Autodesk Fusion 360 part; units mm, degrees
sketch "5.5 drilling alignment tool" plane through (0, 0, 0) normal (0, 1, 0) x (1, 0, 0)
  circle A0 centre (0, 0) radius 2.75
  circle A1 centre (0, 0) radius 4.35
  circle A2 centre (0, 0) radius 21
  line L0 (0, 0) -> (0, 30.5486) construction
  line L1 (0, 0) -> (37.4223, 0) construction
  line L2 (5, 0.7) -> (19, 0.7)
  line L3 (19, 0.7) -> (19, -0.7)
  line L4 (19, -0.7) -> (5, -0.7)
  line L5 (5, -0.7) -> (5, 0.7)
  dimension "d1" = 5.5
  dimension "d2" = 1.6
  dimension "d3" = 42
  dimension "d12" = 5
  dimension "d13" = 14
  dimension "d14" = 1.4
extrude "Extrude1" add sketch "5.5 drilling alignment tool" along normal blind 22 contours A1
extrude "Extrude2" add sketch "5.5 drilling alignment tool" along normal blind 2 contours A2 | L2 L3 L4 L5
chamfer "Chamfer1" distance 2 angle 45 1 edges at (-4.0556, 2, 1.573)
fillet "Fillet1" radius 1 3 faces at (4.3284, 10, 0.4331) (-3.5435, 2.6667, 4.4434) (16.0385, 2, 1.0433)
chamfer "Chamfer2" distance 0.4 angle 45 1 edges at (-19.5789, 0, 7.5939)
extrude "Extrude3" cut sketch "5.5 drilling alignment tool" along normal blind 4 contours L2 L3 L4 L5
pattern_circular "C-Pattern1" count 4 over 360 about axis through (0, 1.75, 0) along (0, 1, 0) of "Extrude3"
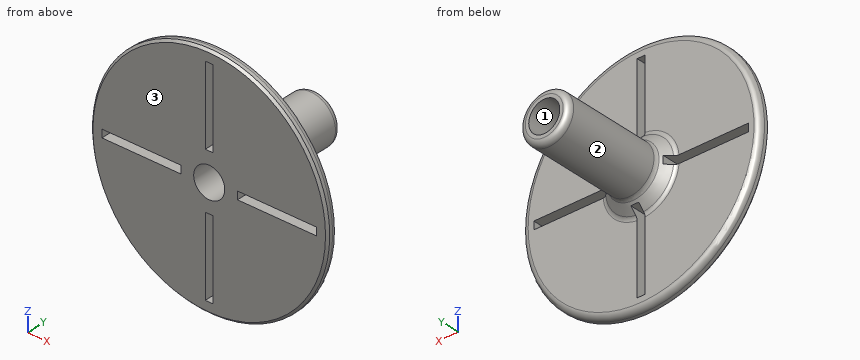
The listing builds one solid part. Answer for the finished solid, in the listing's coordinates (mm). Face numbers are marked on the shaded views. Round coordinates to 2 decimals unless told otherwise and drop trailing zeros. Write each loop counter-clockwise with the first axis right and the second up, starting at its lowest first coordinate (ties: lowest second). Pieces come first, ordered by that corner, then holes. Notation, with made-up numbers: (34.5, 37) -> (62.5, 37) arc R23 cw to (62.5, 63) -> close; hole circle Ø10 at (44.5, 55). An arc over 180 degrees is marked (long way). Use CSV: the item, a comma, the result in double quotes. Start each with the question number.
(1) Section A-A on x = 0 is taken. Count the separate pieces of the cut face and the enclosed holes in it, then the cut area to 3 significant figures.
(2) Consider L1, parallel to Z at x = 0, y = 12; L2, parallel to Y at x = 4, z = 9. Determine where each line is inside the solid, lowest interval first. Write a range as from..to.
(3) The mould has two halves that part along Z. Classify the marked faces 1, 2 and 3: released by +Z, released by -Z, zero draft, split by the parting line, or undercut.
(4) Each of these flat-tipped pins is pushed along its axis until it touches: pin 1 (2.5 mm diameter, centred on x = 9, y = 1.5, fed in from +Z); pin 2 (3 mm diameter, centred on y = 18.5, z = 2, fed in from -X); pin 3 (1 mm diameter, centred on y = 2, z = -13.5, fed in from -X). Where does it stop, or does it pass through?
(5) Section B-B on y = 5.5 is taken. Give the vertices of the cut face in (x, z).
A:
1,separate pieces,"4"
1,enclosed holes,"0"
1,area,"82.2 mm²"
2,L1,"z = -4.35..-2.75, 2.75..4.35"
2,L2,"y = 0..2"
3,face 1,"undercut"
3,face 2,"split by the parting line"
3,face 3,"zero draft"
4,pin 1,"stops at z = 19.49"
4,pin 2,"stops at x = -4.32"
4,pin 3,"stops at x = -16.08"
5,outline,"circle Ø8.7 at (0, 0); hole circle Ø5.5 at (0, 0)"
